Check sheet for the modelled part. Datum: model origin and axes. Units: mm. Give positions to 0.01 mm unless a question says otherwise; leave off trailing zeros. Write each loop counter-clockwise with the first axis right and the second up, starting at its lowest first coordinate (ties: lowest second). Pieces come first, ordered by that corner, then holes. Notation, with made-up numbers: (-8.5, -39) -> (27.5, -39) arc R7 cw to (27.5, -28) -> close; hole circle Ø11 at (9, -5). An arc over 180 degrees is marked (long way). Write each question's results on one line, items separated by ' | '. Start each with the question number.
```python
from build123d import *

# Parameters (mm, degrees)
SKETCH1_W           = 24
SKETCH1_H           = 32
BOSS_EXTRUDE1_DEPTH = 3.5
HOLE1_D             = 7
HOLE1_DEPTH         = 12
HOLE1_CSINK_D       = 9
HOLE1_CSINK_ANGLE   = 60


with BuildPart() as part:
    # Sketch1 → Boss-Extrude1 (new body, symmetric)
    with BuildSketch(Plane.XY):
        Rectangle(SKETCH1_W, SKETCH1_H)
    extrude(amount=BOSS_EXTRUDE1_DEPTH, both=True)

    # Hole1
    with Locations(Plane.XY.offset(3.5)):
        with Locations((0, 8), (0, -8)):
            CounterSinkHole(HOLE1_D / 2, HOLE1_CSINK_D / 2, depth=HOLE1_DEPTH, counter_sink_angle=HOLE1_CSINK_ANGLE)


solid = part.part
```
Item 1: Section check B-B on y = 8. Record the boundary of the cut face in (x, z), then the cut area to 3 significant figures.
Item 2: Section check C-C on z = -2.75. Record the boundary of the cut face in (x, y), then the cut area to 3 significant figures.
Item 3: Depth check by flat-ended pin: pin 1 Ø6.5 at (x, y) = (0, 8) entering from -Z; pin 2 Ø8 at (x, y) = (0, -8) entering from +Z. Enter the tip coordinate at first touch or a pass-through.
Item 4: Section check D-D on x = 2.5. Count the separate pieces of the cut face and the enclosed holes in it, then the cut area to 3 significant figures.
Item 5: Section check A-A on x = 0. Record the boundary of the cut face in (y, z), then the cut area to 3 significant figures.
Item 6: Thickness scan on probe 1 along Y at (x, z) = (0, -1.95); probe 2 along X at (y, z) = (8, -0.3); probe 3 along Y at (x, z) = (-2.5, 1.25). Record the ranges inside material, lowest first. Write a range as from..to.
Check sheet entries:
1) outline: (-12, -3.5) -> (-3.5, -3.5) -> (-3.5, 1.77) -> (-4.5, 3.5) -> (-12, 3.5) -> close; (3.5, -3.5) -> (12, -3.5) -> (12, 3.5) -> (4.5, 3.5) -> (3.5, 1.77) -> close | area: 117 mm^2
2) outline: (-12, -16) -> (12, -16) -> (12, 16) -> (-12, 16) -> close; hole circle Ø7 at (0, -8); hole circle Ø7 at (0, 8) | area: 691 mm^2
3) pin 1: passes through | pin 2: stops at z = 2.63
4) separate pieces: 3 | enclosed holes: 0 | area: 151 mm^2
5) outline: (-16, -3.5) -> (-11.5, -3.5) -> (-11.5, 1.77) -> (-12.5, 3.5) -> (-16, 3.5) -> close; (-4.5, -3.5) -> (4.5, -3.5) -> (4.5, 1.77) -> (3.5, 3.5) -> (-3.5, 3.5) -> (-4.5, 1.77) -> close; (11.5, -3.5) -> (16, -3.5) -> (16, 3.5) -> (12.5, 3.5) -> (11.5, 1.77) -> close | area: 123 mm^2
6) probe 1: y = -16..-11.5, -4.5..4.5, 11.5..16 | probe 2: x = -12..-3.5, 3.5..12 | probe 3: y = -16..-10.45, -5.55..5.55, 10.45..16
